Autodesk Inventor part; units mm, degrees
ref_plane "YZ Plane" through (0, 0, 0) normal (1, 0, 0) x (0, 1, 0)
ref_plane "XZ Plane" through (0, 0, 0) normal (0, 1, 0) x (-1, 0, 0)
ref_plane "XY Plane" through (0, 0, 0) normal (0, 0, 1) x (1, 0, 0)
sketch "Sketch1" plane through (0, 0, 0) normal (0, 0, 1) x (1, 0, 0)
  circle A0 centre (0, 0) radius 55.075
  circle A1 centre (0, 0) radius 75.075
  circle A2 centre (0, 65.075) radius 4
  circle A3 centre (-56.3566, -32.5375) radius 4
  circle A4 centre (56.3566, -32.5375) radius 4
  line L0 (0, 65.075) -> (-56.3566, -32.5375) construction
  line L1 (-56.3566, -32.5375) -> (56.3566, -32.5375) construction
  line L2 (56.3566, -32.5375) -> (0, 65.075) construction
  line L3 (0, 65.075) -> (0, 55.075) construction
  line L4 (-56.3566, -32.5375) -> (-47.6963, -27.5375) construction
  line L5 (56.3566, -32.5375) -> (47.6963, -27.5375) construction
  dimension "d0" = 20
  dimension "d1" = 110.15
  dimension "d7" = 8
  dimension "d8" = 10
extrude "Extrusion1" add sketch "Sketch1" along normal blind 12
properties part number "Tractor_Mobile_2"
Model file for the job. Use its own axes, mm. Coordinates: 2 decimals unless noted, no trailing zeros. Loops run counter-clockwise (first coordinate to the right, second up) from the corner with the lowest first, then second, coordinate; pieces in that order, holes last. Notation, with made-up numbers: (12.25, 35.5) -> (62.25, 35.5) arc R23 ccw to (62.25, 52.5) -> close; hole circle Ø2 at (-8, 55.25). An arc over 180 degrees is marked (long way). Use one line per item in the form item = value. Start each with the question number.
(1) Pull direction X, two halves, no side cores. Call faces 1 (the cylindrical face through (60.17, -33.74, 5.92)), 2 (the cylindrical face through (34.643, 66.604, 5.916)), 3 (the flat face through (0, 56, 12)): pulls with the +X half, pulls with the -X half, needs draft (parallel to the pull), parting line crosses it, or undercut.
(2) Probe probe 1 along Y at (x, z) = (0, 6.25) (3 decimals); probe 2 along Y at (x, z) = (1, 10); probe 3 along X at (y, z) = (-39.5, 9.25). List the from-to ranges inside material, lowest first. Write a range as from..to.
(3) Flat gauge pins, fed straight in: pin 1 (1 mm diameter, centred on x = -23, z = 10.5, fed in from -Y); pin 2 (10.5 mm diameter, centred on x = 0, y = 65.075, fed in from -Z); pin 3 (3 mm diameter, centred on y = 14.5, z = 6.5, fed in from -X); pin 4 (2 mm diameter, centred on y = 45.5, z = 7.5, fed in from +X). Where does each tip first touch, or does it go through?
(4) Cut at A-A on x = 0. Give the cut face in (y, z) (3 decimals).
(5) Cut at C-C on x = -44. Give the cut face in (y, z), and give its area (3 significant figures).
(6) Cut at B-B on y = 0. Give the cut face in (x, z) (3 decimals), and give its area (3 significant figures).
(7) Cut at D-D on z = 4.25. Give the number of separate pieces and of enclosed holes in the cut face, and give its area (3 significant figures).
Values:
q1.face_1 = undercut
q1.face_2 = parting line crosses it
q1.face_3 = needs draft
q2.probe_1 = -75.075..-55.075, 55.075..61.075, 69.075..75.075
q2.probe_2 = -75.07..-55.07, 55.07..61.2, 68.95..75.07
q2.probe_3 = -63.84..-38.38, 38.38..63.84
q3.pin_1 = -71.62
q3.pin_2 = 0
q3.pin_3 = -73.94
q3.pin_4 = 60.46
q4.outline = (-75.075, 0) -> (-55.075, 0) -> (-55.075, 12) -> (-75.075, 12) -> close; (55.075, 0) -> (61.075, 0) -> (61.075, 12) -> (55.075, 12) -> close; (69.075, 0) -> (75.075, 0) -> (75.075, 12) -> (69.075, 12) -> close
q5.outline = (-60.83, 0) -> (-33.12, 0) -> (-33.12, 12) -> (-60.83, 12) -> close; (33.12, 0) -> (60.83, 0) -> (60.83, 12) -> (33.12, 12) -> close
q5.area = 665 mm2
q6.outline = (-75.075, 0) -> (-55.075, 0) -> (-55.075, 12) -> (-75.075, 12) -> close; (55.075, 0) -> (75.075, 0) -> (75.075, 12) -> (55.075, 12) -> close
q6.area = 480 mm2
q7.separate_pieces = 1
q7.enclosed_holes = 4
q7.area = 8,030 mm2
